Here's how the part is built. I have some questions about the finished solid (model axes, mm). Face numbers are marked on the shaded views. Give positions to 0.01 mm unless a question says otherwise; leave off trailing zeros. Loops run counter-clockwise (first coordinate to the right, second up) from the corner with the lowest first, then second, coordinate; pieces in that order, holes last. Notation, with made-up numbers: (49, 49) - (60, 49) arc R23 ccw to (60, 65) - close; hole circle Ø9 at (83.5, 49.5). An arc over 180 degrees is marked (long way). Use one line per item in the form item = value.
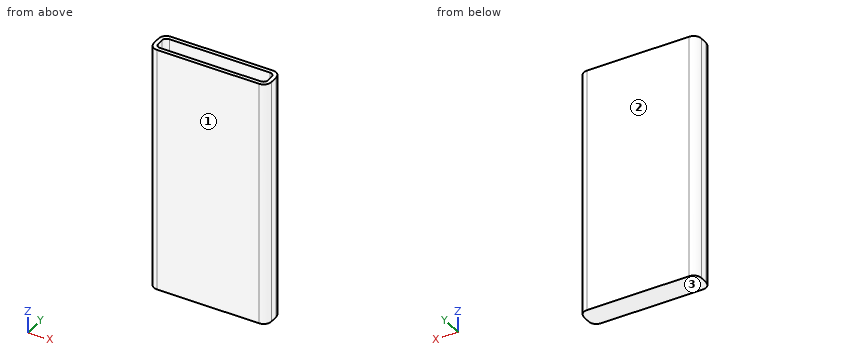
from build123d import *

# Parameters (mm, degrees)
F0_W     = 75
F0_H     = 15
F1_DEPTH = 5
F2_W     = 75
F2_H     = 15
F2_W_2   = 70
F2_H_2   = 10
F3_DEPTH = 160
F4_R     = 5
F5_R     = 5
F6_R     = 5
F7_R     = 5
F8_R     = 3
F9_R     = 3
F10_R    = 3
F11_R    = 3
F12_R    = 3


# Not quite as in the source:
# - two fillets or chamfers of one size are made in one step


with BuildPart() as f1:
    # F0 (on Top) → F1 (new body)
    with BuildSketch(Plane.XY):
        with Locations((-35, 5)):
            Rectangle(F0_W, F0_H)
    extrude(amount=F1_DEPTH)

    # F2 (on face) → F3 (join)
    with BuildSketch(Plane(origin=(0, 0, 0), x_dir=(1, 0, 0), z_dir=(0, 0, -1))):
        with Locations((-35, -5)):
            Rectangle(F2_W, F2_H)
        with Locations((-35, -5)):
            Rectangle(F2_W_2, F2_H_2, mode=Mode.SUBTRACT)
    extrude(amount=-F3_DEPTH)

    # F4
    f4_edges = [f1.edges().sort_by_distance(p)[0] for p in [
        (-72.5, 12.5, 80),
    ]]
    fillet(f4_edges, radius=F4_R)

    # F5
    f5_edges = [f1.edges().sort_by_distance(p)[0] for p in [
        (-72.5, -2.5, 80),
    ]]
    fillet(f5_edges, radius=F5_R)

    # F6
    f6_edges = [f1.edges().sort_by_distance(p)[0] for p in [
        (2.5, -2.5, 80),
    ]]
    fillet(f6_edges, radius=F6_R)

    # F7
    f7_edges = [f1.edges().sort_by_distance(p)[0] for p in [
        (2.5, 12.5, 80),
    ]]
    fillet(f7_edges, radius=F7_R)

    # F8
    f8_edges = [f1.edges().sort_by_distance(p)[0] for p in [
        (-70, 10, 82.5),
    ]]
    fillet(f8_edges, radius=F8_R)

    # F9
    f9_edges = [f1.edges().sort_by_distance(p)[0] for p in [
        (0, 10, 82.5),
    ]]
    fillet(f9_edges, radius=F9_R)

    # F10
    f10_edges = [f1.edges().sort_by_distance(p)[0] for p in [
        (-70, 0, 82.5),
    ]]
    fillet(f10_edges, radius=F10_R)

    # F11
    f11_edges = [f1.edges().sort_by_distance(p)[0] for p in [
        (0, 0, 82.5),
    ]]
    fillet(f11_edges, radius=F11_R)

    # F12
    f12_edges = [f1.edges().sort_by_distance(p)[0] for p in [
        (-35, 0, 5),
        (-0.87868, 0.87868, 5),
        (-69.12132, 0.87868, 5),
        (0, 5, 5),
        (-70, 5, 5),
        (-0.87868, 9.12132, 5),
        (-69.12132, 9.12132, 5),
        (-35, 10, 5),
    ]]
    fillet(f12_edges, radius=F12_R)


solid = f1.part
(1) If we section it at A-A (z = 77.5): List the corners of the cut face in (x, y) for me, plus the area to 3 significant figures.
Geometry says:
outline = (-72.5, 2.5) arc R5 ccw to (-67.5, -2.5) - (-2.5, -2.5) arc R5 ccw to (2.5, 2.5) - (2.5, 7.5) arc R5 ccw to (-2.5, 12.5) - (-67.5, 12.5) arc R5 ccw to (-72.5, 7.5) - close; hole (-70, 3) arc R3 ccw to (-67, 0) - (-3, 0) arc R3 ccw to (0, 3) - (0, 7) arc R3 ccw to (-3, 10) - (-67, 10) arc R3 ccw to (-70, 7) - close
area = 411 mm²
(2) If I drill on probe 1 along X at (y, z) = (5.75, 73.5); probe 2 along Y at (x, z) = (-56, 113.5); probe 3 along Z at (x, y) = (-44, 4), over which ranges is the centre line in solid material (lowest first)?
Geometry says:
probe_1 = -72.5 to -70, 0 to 2.5
probe_2 = -2.5 to 0, 10 to 12.5
probe_3 = 0 to 5
(3) If we section it at B-B (y = 4.5): List the corners of the cut face in (x, z) for me.
Geometry says:
outline = (-72.5, 0) - (2.5, 0) - (2.5, 160) - (0, 160) - (0, 8) arc R3 cw to (-3, 5) - (-67, 5) arc R3 cw to (-70, 8) - (-70, 160) - (-72.5, 160) - close
(4) If we section it at C-C (x = -51): List the corners of the cut face in (y, z) for me, plus the area to 3 significant figures.
Geometry says:
outline = (-2.5, 0) - (12.5, 0) - (12.5, 160) - (10, 160) - (10, 8) arc R3 cw to (7, 5) - (3, 5) arc R3 cw to (0, 8) - (0, 160) - (-2.5, 160) - close
area = 854 mm²
(5) Thinking about a two-plate mould opening in Y: for the marked faces 1, 2 and 3, which applies, pulls with the +Y half, pulls with the -Y half, needs draft (parallel to the pull), parting line crosses it, or undercut?
Geometry says:
face_1 = pulls with the -Y half
face_2 = pulls with the +Y half
face_3 = needs draft
(6) For P1, Ø1.2, axis at x = -43, y = 4.5, coming from the +Z side, with a flat end and sliding along its axis, tell me the tip position at first contact or that it passes through.
Geometry says:
P1 = 5
